```python
from build123d import *

# Parameters (mm, degrees)
SKETCH1_W           = 28
SKETCH1_H           = 10
BOSS_EXTRUDE1_DEPTH = 16
FILLET1_R           = 5


with BuildPart() as part:
    # Sketch1 → Boss-Extrude1 (new, symmetric)
    with BuildSketch(Plane(origin=(0, 0, 0), x_dir=(0, 0, -1), z_dir=(1, 0, 0))):
        Rectangle(SKETCH1_W, SKETCH1_H)
    extrude(amount=BOSS_EXTRUDE1_DEPTH, both=True)

    # Fillet1
    fillet1_edges = [part.edges().sort_by_distance(p)[0] for p in [
        (0, -5, -14),
        (0, -5, 14),
    ]]
    fillet(fillet1_edges, radius=FILLET1_R)


solid = part.part
```
Design review of the part built by this model. Coordinates are the model's own, in mm. Give positions to 0.01 mm unless a question says otherwise; leave off trailing zeros. Loops run counter-clockwise (first coordinate to the right, second up) from the corner with the lowest first, then second, coordinate; pieces in that order, holes last. Notation, with made-up numbers: M 14,-10.5 L 53,-10.5 A13 cw 53,13.5 Z; hole C 78,18 d5. An arc over 180 degrees is marked long. Return JSON: item names as keys, results as strings. Group by question number.
Item 1: For probe 1 along Y at (x, z) = (2, 9.25); probe 2 along Z at (x, y) = (-2.5, -2.75); probe 3 along Y at (x, z) = (3.5, 10), list the stretches that pass through material, from the lowest coordinate up.
Item 2: We need section B-B (y = -3). Give the boundary of the cut face in (x, z), and give its area (3 significant figures).
Item 3: Insertion check: pin 1 Ø3 at (x, y) = (-6, -3) entering from -Z. The pin has a flat end and moves straight along its axis. Give the tip position at first contact, or say it passes through.
Item 4: We need section A-A (x = -8). Give the boundary of the cut face in (y, z), and give its area (3 significant figures).
Output:
{
 "1": {"probe 1": "y = -4.99 to 5", "probe 2": "z = -13.18 to 13.18", "probe 3": "y = -4.9 to 5"},
 "2": {"outline": "M -16,-13 L 16,-13 L 16,13 L -16,13 Z", "area": "832 mm^2"},
 "3": {"pin 1": "stops at z = -13.77"},
 "4": {"outline": "M -5,-9 A5 ccw 0,-14 L 5,-14 L 5,14 L 0,14 A5 ccw -5,9 Z", "area": "269 mm^2"}
}
